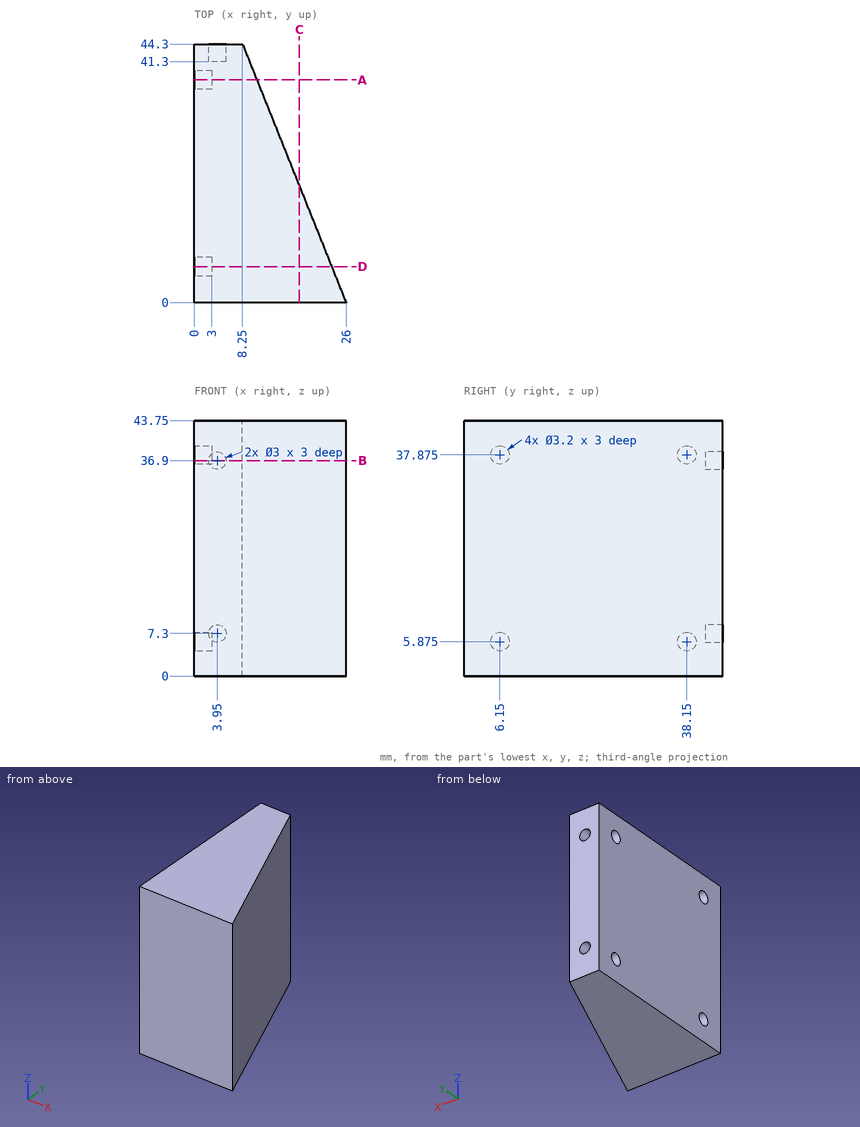
Verification items for this drawing (mm, ordinates from the low corner). Coordinates: 2 decimals unless noted, no trailing zeros. Order: outer loops, then holes, each group sorted by start corner. A loop starts at its lowest first (then second) coordinate and runs counter-clockwise, first axis right, second up. Notation, with made-up numbers: (-31.75, 11.25) - (-17.75, 11.25) arc R17 cw to (-17.75, 35.25) - close; hole circle Ø8 at (74.25, 87). An arc over 180 degrees is marked (long way). Answer in a Markdown table with one row per item. Add a question column.
1. Section check A-A (y = 38.15). Enter the section's corners in (x, z) (3 decimals).
2. Section check C-C (x = 18). Enter the section's corners in (y, z), plus the area to 3 significant figures.
3. Section check B-B (z = 36.9). Enter the section's corners in (x, y), plus the area to 3 significant figures.
4. Material ranges on L1, parallel to Y at x = 19.5, z = 4; L2, parallel to Y at x = 12, z = 7; L3, parallel to X at y = 30.5, z = 40.5, recorded low to high. Write a range as [from, to].
5. Gauge pin test, flat ends, axial feed: pin 1 Ø3 at (y, z) = (6.15, 5.875) entering from +X; pin 2 Ø4 at (y, z) = (11.5, 38.5) entering from +X; pin 3 Ø1.5 at (x, z) = (4, 7.5) entering from +Y. Record the tip position at first contact, or that the pin passes through.
6. Section check D-D (y = 6.15). Enter the section's corners in (x, z) (3 decimals), plus the area to 3 significant figures.
Data:
| question | item | result |
|---|---|---|
| 1 | outline | (0, 0) - (10.714, 0) - (10.714, 43.75) - (0, 43.75) - (0, 39.475) - (3, 39.475) - (3, 36.275) - (0, 36.275) - (0, 7.475) - (3, 7.475) - (3, 4.275) - (0, 4.275) - close |
| 2 | outline | (0, 0) - (19.97, 0) - (19.97, 43.75) - (0, 43.75) - close |
| 2 | area | 874 mm² |
| 3 | outline | (0, 0) - (26, 0) - (8.25, 44.3) - (5.45, 44.3) - (5.45, 41.3) - (2.45, 41.3) - (2.45, 44.3) - (0, 44.3) - (0, 39.42) - (3, 39.42) - (3, 36.88) - (0, 36.88) - (0, 7.42) - (3, 7.42) - (3, 4.88) - (0, 4.88) - close |
| 3 | area | 734 mm² |
| 4 | L1 | y = [0, 16.22] |
| 4 | L2 | y = [0, 34.94] |
| 4 | L3 | x = [0, 13.78] |
| 5 | pin 1 | stops at x = 24.14 |
| 5 | pin 2 | stops at x = 22.19 |
| 5 | pin 3 | stops at y = 41.3 |
| 6 | outline | (0, 0) - (23.536, 0) - (23.536, 43.75) - (0, 43.75) - (0, 39.475) - (3, 39.475) - (3, 36.275) - (0, 36.275) - (0, 7.475) - (3, 7.475) - (3, 4.275) - (0, 4.275) - close |
| 6 | area | 1,010 mm² |
